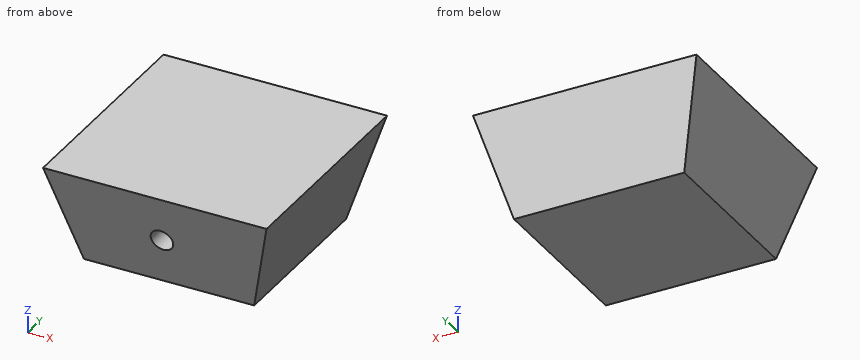
from build123d import *

# Parameters (mm, degrees)
ESQUISSE1_W             = 25.4
ESQUISSE1_H             = 25.4
BOSS_EXTRU_1_DEPTH      = 14.81582
BOSS_EXTRU_1_DRAFT      = -15
ESQUISSE5_R             = 1.666875
ENL_V_MAT_EXTRU_1_DEPTH = 12.7


with BuildPart() as part:
    # Esquisse1 → Boss.-Extru.1 (with draft: the straight prism first)
    with BuildSketch(Plane.XY):
        Rectangle(ESQUISSE1_W, ESQUISSE1_H)
    extrude(amount=BOSS_EXTRU_1_DEPTH)
    # Boss.-Extru.1: the draft: its side faces are tilted about the plane it starts from
    boss_extru_1_sides = [part.faces().sort_by_distance(p)[0] for p in [
        (0, -12.7, 7.40791),
        (12.7, 0, 7.40791),
        (0, 12.7, 7.40791),
        (-12.7, 0, 7.40791),
    ]]
    draft(boss_extru_1_sides, Plane.XY, BOSS_EXTRU_1_DRAFT)

    # Esquisse5 → Enl_v. mat.-Extru.1 (cut)
    with BuildSketch(Plane(origin=(0, -17.78, 0), x_dir=(1, 0, 0), z_dir=(0, 1, 0))):
        with Locations(Location((0, -7.40791, 0), (0, 0, 270))):
            Circle(ESQUISSE5_R)
    extrude(amount=ENL_V_MAT_EXTRU_1_DEPTH, mode=Mode.SUBTRACT)


solid = part.part
Read the model definition and answer for the solid it produces. Units are mm, in the model's axes. Round coordinates to 2 decimals unless told otherwise and drop trailing zeros. Loops run counter-clockwise (first coordinate to the right, second up) from the corner with the lowest first, then second, coordinate; pieces in that order, holes last.
Q1. Section A-A on y = -8 is taken. Write down the section's boundary in (x, z).
Q2. Consider probe 1 along Z at (x, y) = (0, -10); probe 2 along Y at (x, z) = (3.5, 8.75); probe 3 along Y at (x, z) = (9.5, 7). Determine where each line is inside the solid, lowest interval first.
Q3. Section B-B on x = -7.5 is taken. Write down the section's boundary in (y, z), and give its area (3 significant figures).
Q4. Each of these flat-tipped pins is pushed along its axis until it touches: pin 1 (2 mm diameter, centred on y = -12, z = 6.5, fed in from -X); pin 2 (5.5 mm diameter, centred on x = 0, z = 7.41, fed in from -Y); pin 3 (12 mm diameter, centred on x = -10.5, y = -2.5, fed in from -Z); pin 4 (1 mm diameter, centred on x = 10.5, z = 2, fed in from -Y). Where does it stop, or does it pass through?
Q5. Section C-C on z = 6.5 is taken. Write down the section's boundary in (x, y), and give its area (3 significant figures).
Output:
1. outline: (-16.67, 14.82) - (-12.7, 0) - (12.7, 0) - (16.67, 14.82) - close; hole circle Ø3.33 at (0, 7.41)
2. probe 1: z = 0 to 5.74, 9.07 to 14.82
2. probe 2: y = -15.04 to 15.04
2. probe 3: y = -14.58 to 14.58
3. outline: (-16.67, 14.82) - (-12.7, 0) - (12.7, 0) - (16.67, 14.82) - close
3. area: 435 mm2
4. pin 1: stops at x = -14.71
4. pin 2: stops at y = -15.42
4. pin 3: stops at z = 0
4. pin 4: stops at y = -13.37
5. outline: (-14.44, -14.44) - (-1.4, -14.44) - (-1.4, -5.08) - (1.4, -5.08) - (1.4, -14.44) - (14.44, -14.44) - (14.44, 14.44) - (-14.44, 14.44) - close
5. area: 808 mm2
